from build123d import *

# Parameters (mm, degrees)
EXTRUDE_1_DEPTH = 10
FILLET_1_R      = 1
FILLET_2_R      = 3.5


with BuildPart() as part:
    # 草图1 → 凸台-拉伸1 (new body)
    with BuildSketch(Plane(origin=(0, 0, 0), x_dir=(-1, 0, 0), z_dir=(0, 0, -1))):
        Polygon((0, 20), (0, 0), (-15, 0), (-15, 3), (-3, 3), (-3, 20), align=None)
    extrude(amount=-EXTRUDE_1_DEPTH)

    # 圆角1
    fillet_1_edges = [part.edges().sort_by_distance(p)[0] for p in [
        (15, 3, 5),
        (3, 20, 5),
    ]]
    fillet(fillet_1_edges, radius=FILLET_1_R)

    # 圆角2
    fillet_2_edges = [part.edges().sort_by_distance(p)[0] for p in [
        (3, 3, 5),
    ]]
    fillet(fillet_2_edges, radius=FILLET_2_R)


solid = part.part
Can you work these out from the model? Positions are in its coordinate system, mm. A direction names the side the tool comes from. Round coordinates to 2 decimals unless told otherwise and drop trailing zeros. Loops run counter-clockwise (first coordinate to the right, second up) from the corner with the lowest first, then second, coordinate; pieces in that order, holes last. Notation, with made-up numbers: (39, -32) - (64, -32) arc R24 ccw to (64, 7) - close; hole circle Ø6 at (-10.5, 52.25). An arc over 180 degrees is marked (long way). Write item = value, one per line. Start each with the question number.
(1) If we section it at B-B (y = 5.25): Please give me the cut outline in (x, z).
(2) If we section it at A-A (z = 7): Please give me the cut outline in (x, y), and give its area (3 significant figures).
(3) For faces 1 (the face through (10, 3, 5)), 2 (the face through (1, 20, 5)), which set-ups out of +Z, -Z, +X, -X, +Y, -Y let a thin tool reach every point of the face, with its end or its side?
(4) For P1, Ø2, axis at x = 5.5, z = 4.5, coming from the -Y side; P2, Ø5, axis at y = 16, z = 6, coming from the +X side; P3, Ø6, axis at x = 10.5, z = 4, coming from the +Y side, each with a flat end and sliding along its axis, tell me the tip position at first contact or that it passes through.
(5) If I drill on probe 1 along Y at (x, z) = (7.5, 3.5); probe 2 along X at (y, z) = (5.5, 5.5), over which ranges is the centre line in solid material (lowest first)? Write a range as [from, to].
(6) If we section it at C-C (x = 9): Please give me the cut outline in (y, z).
Ans:
q1.outline = (0, 0) - (3.23, 0) - (3.23, 10) - (0, 10) - close
q2.outline = (0, 0) - (15, 0) - (15, 2) arc R1 ccw to (14, 3) - (6.5, 3) arc R3.5 cw to (3, 6.5) - (3, 19) arc R1 ccw to (2, 20) - (0, 20) - close
q2.area = 98.2 mm²
q3.face_1 = +Z, -Z, +X, +Y
q3.face_2 = +Z, -Z, +X, -X, +Y
q4.P1 = 0
q4.P2 = 3
q4.P3 = 3
q5.probe_1 = [0, 3]
q5.probe_2 = [0, 3.15]
q6.outline = (0, 0) - (3, 0) - (3, 10) - (0, 10) - close
